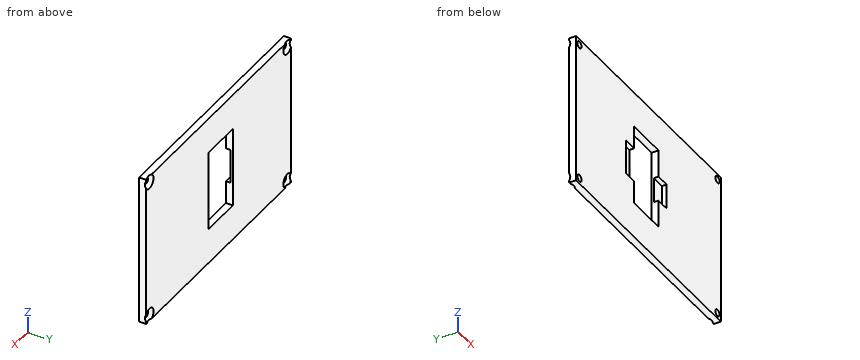
```python
from build123d import *

# Parameters (mm, degrees)
CROQUIS1_W              = 106
CROQUIS1_H              = 66
SALIENTE_EXTRUIR1_DEPTH = 3
CROQUIS2_W              = 17.819535579
CROQUIS2_H              = 35
CORTAR_EXTRUIR1_DEPTH   = 3
CROQUIS3_W              = 6
CROQUIS3_H              = 11
CROQUIS3_H_2            = 15
CORTAR_EXTRUIR2_DEPTH   = 2
CROQUIS4_R              = 1.5
CORTAR_EXTRUIR3_DEPTH   = 4
CHAFL_N1_SIZE           = 1.5


with BuildPart() as part:
    # Croquis1 → Saliente-Extruir1 (new body)
    with BuildSketch(Plane(origin=(0, 0, 0), x_dir=(1, 0, 0), z_dir=(0, 1, 0))):
        with Locations((10.650118203, -3.555555556)):
            Rectangle(CROQUIS1_W, CROQUIS1_H)
    extrude(amount=SALIENTE_EXTRUIR1_DEPTH)

    # Croquis2 → Cortar-Extruir1 (cut)
    with BuildSketch(Plane(origin=(0, 3, 0), x_dir=(1, 0, 0), z_dir=(0, 1, 0))):
        with Locations((9.059885993, -3.555555556)):
            Rectangle(CROQUIS2_W, CROQUIS2_H)
    extrude(amount=-CORTAR_EXTRUIR1_DEPTH, mode=Mode.SUBTRACT)

    # Croquis3 → Cortar-Extruir2 (cut)
    with BuildSketch(Plane.XZ):
        with Locations((20.969653782, 3.555555556)):
            Rectangle(CROQUIS3_W, CROQUIS3_H)
        with Locations((-2.849881797, 3.555555556)):
            Rectangle(CROQUIS3_W, CROQUIS3_H_2)
    extrude(amount=-CORTAR_EXTRUIR2_DEPTH, mode=Mode.SUBTRACT)

    # Croquis4 → Cortar-Extruir3 (cut)
    with BuildSketch(Plane(origin=(0, 3, 0), x_dir=(1, 0, 0), z_dir=(0, 1, 0))):
        with Locations(Location((-39.849881797, 26.944444444, 0), (0, 0, 270))):
            Circle(CROQUIS4_R)
        with Locations(Location((61.150118203, 26.944444444, 0), (0, 0, 270))):
            Circle(CROQUIS4_R)
        with Locations(Location((61.150118203, -34.055555556, 0), (0, 0, 270))):
            Circle(CROQUIS4_R)
        with Locations(Location((-39.849881797, -34.055555556, 0), (0, 0, 270))):
            Circle(CROQUIS4_R)
    extrude(amount=-CORTAR_EXTRUIR3_DEPTH, mode=Mode.SUBTRACT)

    # Chaflán1
    # the kernel refuses this chamfer: 1.5 mm, written as the material it takes off along each edge
    with BuildSketch(Plane(origin=(-39.849881797, 3, 34.055555556), x_dir=(0, 0, 1), z_dir=(-1, 0, 0))) as chafl_n1_piece_1:
        Polygon((1.5 + CHAFL_N1_SIZE, 0), (1.5, -CHAFL_N1_SIZE), (1.5, 0), align=None)
    revolve(axis=Axis((-39.849881797, 3, 34.055555556), (0, 1, 0)), mode=Mode.SUBTRACT)
    with BuildSketch(Plane(origin=(61.150118203, 3, 34.055555556), x_dir=(0, 0, 1), z_dir=(-1, 0, 0))) as chafl_n1_piece_2:
        Polygon((1.5 + CHAFL_N1_SIZE, 0), (1.5, -CHAFL_N1_SIZE), (1.5, 0), align=None)
    revolve(axis=Axis((61.150118203, 3, 34.055555556), (0, 1, 0)), mode=Mode.SUBTRACT)
    with BuildSketch(Plane(origin=(61.150118203, 3, -26.944444444), x_dir=(0, 0, 1), z_dir=(-1, 0, 0))) as chafl_n1_piece_3:
        Polygon((1.5 + CHAFL_N1_SIZE, 0), (1.5, -CHAFL_N1_SIZE), (1.5, 0), align=None)
    revolve(axis=Axis((61.150118203, 3, -26.944444444), (0, 1, 0)), mode=Mode.SUBTRACT)
    with BuildSketch(Plane(origin=(-39.849881797, 3, -26.944444444), x_dir=(0, 0, 1), z_dir=(-1, 0, 0))) as chafl_n1_piece_4:
        Polygon((1.5 + CHAFL_N1_SIZE, 0), (1.5, -CHAFL_N1_SIZE), (1.5, 0), align=None)
    revolve(axis=Axis((-39.849881797, 3, -26.944444444), (0, 1, 0)), mode=Mode.SUBTRACT)


solid = part.part
```
Input: part model. Units: mm. Frame: model coordinates. Give positions to 0.01 mm unless a question says otherwise; leave off trailing zeros. Loops run counter-clockwise (first coordinate to the right, second up) from the corner with the lowest first, then second, coordinate; pieces in that order, holes last.
1) Line query: L1, parallel to X at y = 2.1, z = 7.5; L2, parallel to Z at x = 2, y = 1.8; L3, parallel to Z at x = -4, y = 1.85. Output: solid intervals per line, ascending.
A:
L1: x = -42.35 to 0.15, 17.97 to 63.65
L2: z = -29.44 to -13.94, 21.06 to 36.56
L3: z = -29.44 to -3.94, 11.06 to 36.56
2) Section query A-A on x = 9. Return the cut outline in (y, z), and give its area (3 significant figures).
A:
outline: (0, -29.44) - (3, -29.44) - (3, -13.94) - (0, -13.94) - close; (0, 21.06) - (3, 21.06) - (3, 36.56) - (0, 36.56) - close
area: 93.0 mm2
3) Section query B-B on z = -12. Return the cut outline in (x, y), and give its area (3 significant figures).
A:
outline: (-42.35, 0) - (0.15, 0) - (0.15, 3) - (-42.35, 3) - close; (17.97, 0) - (63.65, 0) - (63.65, 3) - (17.97, 3) - close
area: 265 mm2
4) Section query C-C on y = 0.5. Return the cut outline in (x, z), and give its area (3 significant figures).
A:
outline: (-42.35, -29.44) - (63.65, -29.44) - (63.65, 36.56) - (-42.35, 36.56) - close; hole circle Ø3 at (-39.85, -26.94); hole circle Ø3 at (-39.85, 34.06); hole (-5.85, -3.94) - (0.15, -3.94) - (0.15, -13.94) - (17.97, -13.94) - (17.97, -1.94) - (23.97, -1.94) - (23.97, 9.06) - (17.97, 9.06) - (17.97, 21.06) - (0.15, 21.06) - (0.15, 11.06) - (-5.85, 11.06) - close; hole circle Ø3 at (61.15, -26.94); hole circle Ø3 at (61.15, 34.06)
area: 6,190 mm2
5) Contact query for a flat-ended pin moving along its axis: pin 1 (3 mm diameter, centred on x = 21.5, z = 1, fed in from -Y). Output: stop coordinate, or through.
A:
pin 1: stops at y = 2
